Autodesk Inventor part; units mm, degrees
ref_plane "Plano inicial" through (0, 0, -20) normal (0, 0, 1) x (1, 0, 0)
ref_plane "Plano final" through (0, 0, 120) normal (0, 0, 1) x (1, 0, 0)
ref_plane "Plano de trabalho5" through (15, 0, 120) normal (-0.7071, 0, 0.7071) x (0.7071, 0, 0.7071)
ref_plane "Plano inicial" through (0, 0, -20) normal (0, 0, 1) x (1, 0, 0)
ref_plane "Plano final" through (0, 0, 120) normal (0, 0, 1) x (1, 0, 0)
sketch "Esboço" plane through (0, 0, 0) normal (0, 0, 1) x (1, 0, 0)
  line L0 (-15, -21) -> (-15, 21)
  line L1 (-11, 25) -> (11, 25)
  line L2 (15, 21) -> (15, -21)
  line L3 (11, -25) -> (-11, -25)
  arc A0 (-15, -21) -> (-11, -25) centre (-11, -21) ccw
  arc A1 (15, 21) -> (11, 25) centre (11, 21) ccw
  arc A2 (-11, 25) -> (-15, 21) centre (-11, 21) ccw
  arc A3 (11, -25) -> (15, -21) centre (11, -21) ccw
  arc A4 (-11, 23) -> (-13, 21) centre (-11, 21) ccw
  line L4 (-11, 23) -> (11, 23)
  arc A5 (13, 21) -> (11, 23) centre (11, 21) ccw
  line L5 (13, 21) -> (13, -21)
  arc A6 (11, -23) -> (13, -21) centre (11, -21) ccw
  line L6 (11, -23) -> (-11, -23)
  arc A7 (-13, -21) -> (-11, -23) centre (-11, -21) ccw
  line L7 (-13, -21) -> (-13, 21)
  line L8 (0, 36.1598) -> (0, -36.1598) construction
  line L9 (-22.1598, 0) -> (22.1598, 0) construction
  dimension "d7" = 4
  dimension "d9" = 30
  dimension "d11" = 50
  dimension "d12" = 2
  dimension "d15" = 15
  dimension "d16" = 25
extrude "Corpo" add sketch "Esboço" along normal up to surface (140 mm away) from surface at -20
sketch "Sketch3" plane through (0, 0, 0) normal (0, 0, 1) x (1, 0, 0)
  line L0 (0, 0) -> (10, 0)
ref_plane "Work Plane3" through (0, 0, 0) normal (0, -1, 0) x (1, 0, 0)
sketch "Sketch4" plane through (0, 0, 0) normal (0, -1, 0) x (1, 0, 0)
  line L0 (-2, -20) -> (12, -20)
  line L1 (-2, 120) -> (12, 120)
  dimension "d18" = 140
ref_plane "Plano de trabalho5" through (15, 0, 120) normal (-0.7071, 0, 0.7071) x (0.7071, 0, 0.7071)
split "Dividir2" plane through (15, 0, 120) removes the side toward (-0.7071, 0, 0.7071)
ref_plane "Plano de trabalho6" through (15, 0, -20) normal (-0.5547, 0, -0.8321) x (-0.8321, 0, 0.5547)
split "Dividir3" plane through (15, 0, -20) removes the side toward (-0.5547, 0, -0.8321)
equation "\"d7\" = G_IR"
equation "\"d9\" = G_W"
equation "\"d11\" = G_H"
equation "\"d12\" = G_T"
equation "\"d15\" = 0.5 * d9"
equation "\"d16\" = 0.5 * d11"
equation "\"d3\" = G_L"
equation "\"G_W\" = 30"
equation "\"G_H\" = 50"
equation "\"G_T\" = 2"
equation "\"G_IR\" = 4"
equation "\"G_L\" = d18"
equation "\"G_OFFSET_END\" = 30"
equation "\"d14\" = G_OFFSET_END + B_L"
equation "\"B_L\" = 90"
properties part number "ISO 4019 - 50x30x2 - 140" material "Aço, suave"
Work out the finished part from the listing and answer in its coordinate system (mm). A direction names the side the tool comes from. Give positions to 0.01 mm unless a question says otherwise; leave off trailing zeros. Order: outer loops, then holes, each group sorted by start corner. A loop starts at its lowest first (then second) coordinate and runs counter-clockwise, first axis right, second up. Notation, with made-up numbers: (53, 53.25) - (109, 53.25) arc R15 cw to (109, 81.25) - close; hole circle Ø2 at (-8.5, -7). An arc over 180 degrees is marked (long way). Answer as CSV lines item,"result". Start each with the question number.
Q1. The part is cut by section C-C (x = -2). Write down the section's boundary in (y, z), then the cut area to 3 significant figures.
Q2. The part is cut by section A-A (y = -2.5). Write down the section's boundary in (x, z).
Q3. For faces 1 (the face through (0, -23, 48)), 2 (the face through (13.859, -23.797, 49.02)), determine the directions among +Z, -Z, +X, -X, +Y, -Y from which every point of the face is accessible in a straight line to the end or side of a thin tool.
Q4. The mould has two halves that part along Y. Classify faces 3 (the face through (13.26, 1.97, -18.84)), 4 (the face through (-13.859, 23.797, 44.989)), 5 (the face through (-13, 0, 45)): +Y half, -Y half, draft (parallel to the pull), parting line (faces both ways), or undercut.
Q5. Find the intervals of material crossed by L1, parallel to Y at x = -7.5, z = 26; L2, parallel to X at y = -5, z = 55; L3, parallel to X at y = -4, z = -8.5, in increasing order. Write a range as [from, to].
Q6. The part is cut by section B-B (z = 13). Write down the section's boundary in (x, y).
Check result:
1,outline,"(-25, -8.67) - (-23, -8.67) - (-23, 103) - (-25, 103) - close; (23, -8.67) - (25, -8.67) - (25, 103) - (23, 103) - close"
1,area,"447 mm²"
2,outline,"(-15, 0) - (-13, -1.33) - (-13, 92) - (-15, 90) - close; (13, -18.67) - (15, -20) - (15, 120) - (13, 118) - close"
3,face 1,"+Z, -Z"
3,face 2,"+Z, -Z, +X, -Y"
4,face 3,"draft"
4,face 4,"+Y half"
4,face 5,"undercut"
5,L1,"y = [-25, -23], [23, 25]"
5,L2,"x = [-15, -13], [13, 15]"
5,L3,"x = [13, 15]"
6,outline,"(-15, -21) arc R4 ccw to (-11, -25) - (11, -25) arc R4 ccw to (15, -21) - (15, 21) arc R4 ccw to (11, 25) - (-11, 25) arc R4 ccw to (-15, 21) - close; hole (-13, -21) arc R2 ccw to (-11, -23) - (11, -23) arc R2 ccw to (13, -21) - (13, 21) arc R2 ccw to (11, 23) - (-11, 23) arc R2 ccw to (-13, 21) - close"
